from build123d import *

# Parameters (mm, degrees)
F0_W     = 60
F0_H     = 30
F1_DEPTH = 25
F2_R     = 3.2
F3_T     = -1.6
F4_W     = 1.6
F4_H     = 26.8
F5_DEPTH = 23.4
F6_R     = 1.6
F7_R     = 1.6


with BuildPart() as f1:
    # F0 (on Top) → F1 (new body)
    with BuildSketch(Plane.XY):
        Rectangle(F0_W, F0_H)
    extrude(amount=F1_DEPTH)

    # F2
    f2_edges = [f1.edges().sort_by_distance(p)[0] for p in [
        (-30, 15, 12.5),
        (-30, -15, 12.5),
        (30, -15, 12.5),
        (30, 15, 12.5),
    ]]
    fillet(f2_edges, radius=F2_R)

    # F3
    f3_openings = [f1.faces().sort_by_distance(p)[0] for p in [
        (0, 0, 25),
    ]]
    offset(amount=F3_T, openings=f3_openings)

    # F4 (on face) → F5 (join, through all)
    with BuildSketch(Plane.XY.offset(25)):
        Rectangle(F4_W, F4_H)
    extrude(amount=-F5_DEPTH)

    # F6
    f6_edges = [f1.edges().sort_by_distance(p)[0] for p in [
        (-0.8, 13.4, 13.3),
        (0.8, 13.4, 13.3),
        (-0.8, -13.4, 13.3),
        (0.8, -13.4, 13.3),
    ]]
    fillet(f6_edges, radius=F6_R)

    # F7
    f7_edges = [f1.edges().sort_by_distance(p)[0] for p in [
        (-14.6, 13.4, 1.6),
        (14.6, 13.4, 1.6),
    ]]
    fillet(f7_edges, radius=F7_R)


solid = f1.part
The listing builds one solid part. Answer for the finished solid, in the listing's coordinates (mm). A direction names the side the tool comes from. Round coordinates to 2 decimals unless told otherwise and drop trailing zeros. Write each loop counter-clockwise with the first axis right and the second up, starting at its lowest first coordinate (ties: lowest second). Pieces come first, ordered by that corner, then holes. Notation, with made-up numbers: M -34.75,-15 L -6.75,-15 A21 cw -6.75,-6 Z; hole C 8.25,13.5 d11. An arc over 180 degrees is marked long. Write each question's results on one line, items separated by ' | '. Start each with the question number.
Item 1: Find section A-A on z = 13. Write down the section's boundary in (x, y), and give its area (3 significant figures).
Item 2: Which of the six approach directions +Z, -Z, +X, -X, +Y, -Y give full straight-line access (tool end or side, diameter ignored) to faces 5 (the cylindrical face through (27.94, 12.92, 14.25)), 6 (the cylindrical face through (-29.087, -14.038, 12.675))?
Item 3: The mould has two halves that part along Y. Classify faces 1 (the cylindrical face through (29.087, 14.038, 12.675)), 2 (the flat face through (0, 0, 0)), 3 (the cylindrical face through (-1.26, -0.17, 2.08)), 4 (the flat face through (-15, -13.4, 14)): +Y half, -Y half, draft (parallel to the pull), parting line (faces both ways), or undercut.
Item 4: Straight lines are drawn through the part: probe 1 along X at (y, z) = (9.25, 22.75); probe 2 along Y at (x, z) = (-12, 15.25); probe 3 along Z at (x, y) = (-12.5, 10.5). For each, find the intervals that lie inside material, in ascending order.
Item 5: Find section C-C on y = -1.75. Write down the section's boundary in (x, z), and give its area (3 significant figures).
Item 6: Find section B-B on x = -22. Write down the section's boundary in (y, z), and give its area (3 significant figures).
Item 7: Find section D-D on x = -1.5. Write down the section's boundary in (y, z).
Item 8: Given pin 1 Ø5 at (x, y) = (-13, -9) entering from +Z; pin 2 Ø1.5 at (x, y) = (-9, -11.5) entering from +Z, each flat-ended and moving along its own axis, determine where each tip first touches the part or whether it passes through.
Answer block:
1) outline: M -30,-11.8 A3.2 ccw -26.8,-15 L 26.8,-15 A3.2 ccw 30,-11.8 L 30,11.8 A3.2 ccw 26.8,15 L -26.8,15 A3.2 ccw -30,11.8 Z; hole M -28.4,-11.8 A1.6 ccw -26.8,-13.4 L -2.4,-13.4 A1.6 ccw -0.8,-11.8 L -0.8,11.8 A1.6 ccw -2.4,13.4 L -26.8,13.4 A1.6 ccw -28.4,11.8 Z; hole M 0.8,-11.8 A1.6 ccw 2.4,-13.4 L 26.8,-13.4 A1.6 ccw 28.4,-11.8 L 28.4,11.8 A1.6 ccw 26.8,13.4 L 2.4,13.4 A1.6 ccw 0.8,11.8 Z | area: 316 mm²
2) face 5: +Z | face 6: +Z, -Z, -X, -Y
3) face 1: +Y half | face 2: draft | face 3: undercut | face 4: undercut
4) probe 1: x = -30 to -28.4, -0.8 to 0.8, 28.4 to 30 | probe 2: y = -15 to -13.4, 13.4 to 15 | probe 3: z = 0 to 1.6
5) outline: M -30,0 L 30,0 L 30,25 L 28.4,25 L 28.4,3.2 A1.6 cw 26.8,1.6 L 2.4,1.6 A1.6 cw 0.8,3.2 L 0.8,25 L -0.8,25 L -0.8,3.2 A1.6 cw -2.4,1.6 L -26.8,1.6 A1.6 cw -28.4,3.2 L -28.4,25 L -30,25 Z | area: 211 mm²
6) outline: M -15,0 L 15,0 L 15,25 L 13.4,25 L 13.4,3.2 A1.6 cw 11.8,1.6 L -11.8,1.6 A1.6 cw -13.4,3.2 L -13.4,25 L -15,25 Z | area: 124 mm²
7) outline: M -15,0 L 15,0 L 15,25 L 13.12,25 L 13.12,3.2 A1.32 cw 11.8,1.88 L -11.8,1.88 A1.32 cw -13.12,3.2 L -13.12,25 L -15,25 Z
8) pin 1: stops at z = 1.6 | pin 2: stops at z = 1.66
